from build123d import *

# Parameters (mm, degrees)
SUPERFICIE_EXTRUIR1_1_DEPTH = 1060
DAR_ESPESOR1_T2             = 1


with BuildPart() as body_1:
    # Superficie-Extruir1: a surface, the sketch's curves swept straight by 1060 mm
    with BuildLine(Plane.XY, mode=Mode.PRIVATE) as superficie_extruir1_1_path:
        Line((0, 0), (-40, 0))
        Line((-40, 0), (-40, 40))
    superficie_extruir1_1 = Shell.extrude(superficie_extruir1_1_path.wire(), (0 * SUPERFICIE_EXTRUIR1_1_DEPTH, 0 * SUPERFICIE_EXTRUIR1_1_DEPTH, 1 * SUPERFICIE_EXTRUIR1_1_DEPTH))
    add(Solid.thicken(superficie_extruir1_1, -DAR_ESPESOR1_T2))


solid = body_1.part
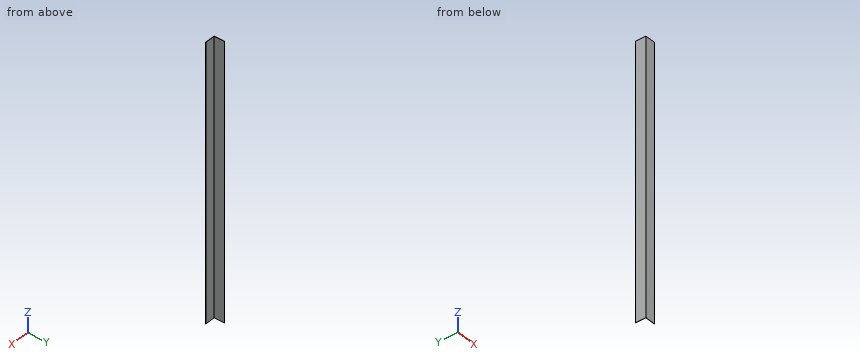
The listing builds one solid part. Answer for the finished solid, in the listing's coordinates (mm). Coordinates: 2 decimals unless noted, no trailing zeros. Write each loop counter-clockwise with the first axis right and the second up, starting at its lowest first coordinate (ties: lowest second). Pieces come first, ordered by that corner, then holes. Notation, with made-up numbers: (79, 63) -> (85, 63) arc R25 ccw to (85, 81) -> close; hole circle Ø9 at (46.25, -17.75). An arc over 180 degrees is marked (long way). One line per question, with ' | ' between items.
1. Section A-A (z = 352.5) is taken. Determine the outline of the cut face in (x, y).
Verdict:
outline: (-40, 0) -> (0, 0) -> (0, 1) -> (-39, 1) -> (-39, 40) -> (-40, 40) -> close
2. Section C-C (x = -30) is taken. Determine the outline of the cut face in (y, z), and give its area (3 significant figures).
Verdict:
outline: (0, 0) -> (1, 0) -> (1, 1060) -> (0, 1060) -> close | area: 1,060 mm^2
3. Section B-B (y = 23.5) is taken. Determine the outline of the cut face in (x, z), and give its area (3 significant figures).
Verdict:
outline: (-40, 0) -> (-39, 0) -> (-39, 1060) -> (-40, 1060) -> close | area: 1,060 mm^2
4. Given pin 1 Ø10 at (x, z) = (-32, 429) entering from +Y; pin 2 Ø8 at (y, z) = (25, 802.5) entering from +X, each flat-ended and moving along its own axis, determine where each tip first touches the part or whether it passes through.
Verdict:
pin 1: stops at y = 1 | pin 2: stops at x = -39
5. Straight lines are drawn through the part: line 1 (X direction, y = 11, z = 58.5); line 2 (Y direction, x = -8.5, z = 400.5). For each, find the intervals that lie inside material, in ascending order.
Verdict:
line 1: x = -40 to -39 | line 2: y = 0 to 1
